```python
from build123d import *

# Parameters (mm, degrees)
F0_R      = 12
F1_DEPTH  = 1
F3_DEPTH  = 1
F4_R      = 1.5
F5_DEPTH  = 25
F6_SIZE   = 0.5
F7_R      = 6.35
F8_DEPTH  = 25
F9_R      = 1.5
F10_DEPTH = 25
F11_SIZE  = 0.5


with BuildPart() as f1:
    # F0 (on Front) → F1 (new body)
    with BuildSketch(Plane.XZ):
        with BuildLine():
            ThreePointArc((64.5, -22.5), (87, 0), (64.5, 22.5))
            Line((64.5, 22.5), (-64.5, 22.5))
            ThreePointArc((-64.5, 22.5), (-87, 0), (-64.5, -22.5))
            Line((-64.5, -22.5), (64.5, -22.5))
        make_face()
        with Locations((-64.5, 0)):
            Circle(F0_R, mode=Mode.SUBTRACT)
        with Locations((64.5, 0)):
            Circle(F0_R, mode=Mode.SUBTRACT)
    extrude(amount=F1_DEPTH)

    # F2 (on face) → F3 (join)
    with BuildSketch(Plane.XZ.offset(1)):
        Polygon((-87, -22.5), (-64.5, -22.5), (-64.5, -17.4313578755), (-70.5482587218, -14.7617282346), (-78.2682448626, -9.4630774111), (-80.8771923184, 0), (-87, 0), align=None)
    extrude(amount=-F3_DEPTH)

    # F4 (on face) → F5 (cut)
    with BuildSketch(Plane.XZ.offset(1)):
        with Locations((-53.5, 16)):
            Circle(F4_R)
        with Locations((-53.5, -16)):
            Circle(F4_R)
        with Locations((53.5, 16)):
            Circle(F4_R)
        with Locations((53.5, -16)):
            Circle(F4_R)
    extrude(amount=-F5_DEPTH, mode=Mode.SUBTRACT)

    # F6
    f6_edges = [f1.edges().sort_by_distance(p)[0] for p in [
        (-55, 0, 16),
        (-55, 0, -16),
        (52, 0, 16),
        (52, 0, -16),
    ]]
    chamfer(f6_edges, length=F6_SIZE)

    # F7 (on face) → F8 (cut)
    with BuildSketch(Plane.XZ.offset(1)):
        Circle(F7_R)
    extrude(amount=-F8_DEPTH, mode=Mode.SUBTRACT)

    # F9 (on face) → F10 (cut)
    with BuildSketch(Plane.XZ.offset(1)):
        with Locations((-11.35, 4)):
            Circle(F9_R)
        with Locations((-11.35, -4)):
            Circle(F9_R)
        with Locations((11.35, 4)):
            Circle(F9_R)
        with Locations((11.35, -4)):
            Circle(F9_R)
    extrude(amount=-F10_DEPTH, mode=Mode.SUBTRACT)

    # F11
    f11_edges = [f1.edges().sort_by_distance(p)[0] for p in [
        (-12.85, 0, 4),
        (-12.85, 0, -4),
        (9.85, 0, -4),
        (9.85, 0, 4),
    ]]
    chamfer(f11_edges, length=F11_SIZE)


solid = f1.part
```
Can you work these out from the model? Positions are in its coordinate system, mm. Give positions to 0.01 mm unless a question says otherwise; leave off trailing zeros. Write each loop counter-clockwise with the first axis right and the second up, starting at its lowest first coordinate (ties: lowest second). Pieces come first, ordered by that corner, then holes. Notation, with made-up numbers: (11, 50) -> (49, 50) arc R22 cw to (49, 89) -> close; hole circle Ø2 at (66, 69). An arc over 180 degrees is marked (long way). Write item = value, one per line.
(1) Suppose I cut it at D-D on z = 16. Write out the boundary of the cut face in (x, y).
Worked out:
outline = (-80.32, -1) -> (-55, -1) -> (-55, -0.5) -> (-55.5, 0) -> (-80.32, 0) -> close; (-52, -1) -> (52, -1) -> (52, -0.5) -> (51.5, 0) -> (-51.5, 0) -> (-52, -0.5) -> close; (55, -1) -> (80.32, -1) -> (80.32, 0) -> (55.5, 0) -> (55, -0.5) -> close
(2) Suppose I cut it at B-B on z = -4. Write out the boundary of the cut face in (x, y).
Worked out:
outline = (-87, -1) -> (-75.81, -1) -> (-75.81, 0) -> (-87, 0) -> close; (-53.19, -1) -> (-12.85, -1) -> (-12.85, -0.5) -> (-13.35, 0) -> (-53.19, 0) -> close; (-9.85, -1) -> (-4.93, -1) -> (-4.93, 0) -> (-9.35, 0) -> (-9.85, -0.5) -> close; (4.93, -1) -> (9.85, -1) -> (9.85, -0.5) -> (9.35, 0) -> (4.93, 0) -> close; (12.85, -1) -> (53.19, -1) -> (53.19, 0) -> (13.35, 0) -> (12.85, -0.5) -> close; (75.81, -1) -> (86.64, -1) -> (86.64, 0) -> (75.81, 0) -> close
(3) Suppose I cut it at A-A on y = -0.3. Count the separate pieces of the cut face and the enclosed holes in it, then the cut area to 3 significant figures.
Worked out:
separate_pieces = 1
enclosed_holes = 11
area = 6,400 mm^2
(4) Suppose I cut it at C-C on x = -69.5. Write out the boundary of the cut face in (y, z).
Worked out:
outline = (-1, -22.5) -> (0, -22.5) -> (0, -10.91) -> (-1, -10.91) -> close; (-1, 10.91) -> (0, 10.91) -> (0, 21.94) -> (-1, 21.94) -> close
(5) Thinking about a two-plate mould opening in Z: for faces 1 (the face through (-80.234, -0.493, 16.084)), 2 (the face through (52.3, -0.8, -16.9)), 3 (the face through (-1, -1, -10)), which applies, released by +Z, released by -Z, zero draft, split by the parting line, or undercut?
Worked out:
face_1 = released by +Z
face_2 = undercut
face_3 = zero draft
(6) I'm going to push a flat-ended pin straight in: P1, Ø5, axis at x = 11.35, z = 4, coming from the -Y side. Where does the tip first touch, or does it pass through?
Worked out:
P1 = -1
(7) I need wall thicknesses on probe 1 along Z at (x, y) = (11.35, -0.7); probe 2 along Z at (x, y) = (2, -0.35); probe 3 along Z at (x, y) = (-64.5, -0.65). Which ranges of each line are inside material? Lowest first, please. Write a range as from..to.
Worked out:
probe_1 = -22.5..-5.5, -2.5..2.5, 5.5..22.5
probe_2 = -22.5..-6.03, 6.03..22.5
probe_3 = -22.5..-12, 12..22.5
